Verification items for the finished model (mm, model axes). A direction names the side the tool comes from. Give positions to 0.01 mm unless a question says otherwise; leave off trailing zeros. Write each loop counter-clockwise with the first axis right and the second up, starting at its lowest first coordinate (ties: lowest second). Pieces come first, ordered by that corner, then holes. Notation, with made-up numbers: (10, -8.75) - (17, -8.75) arc R23 cw to (17, 27.25) - close; hole circle Ø7 at (54.5, -19). An arc over 180 degrees is marked (long way). Put each result on its own line as item: value.
from build123d import *

# Parameters (mm, degrees)
SKETCH1_R           = 30
SKETCH1_R_2         = 12
SKETCH1_R_3         = 20
BOSS_EXTRUDE1_DEPTH = 50
FILLET1_R           = 6
FILLET2_R           = 5


with BuildPart() as part:
    # Sketch1 → Boss-Extrude1 (new body)
    with BuildSketch(Plane.XY):
        with BuildLine():
            Line((0, 0), (168, 0))
            Line((168, 0), (168, 24))
            Line((168, 24), (134, 24))
            Line((134, 24), (134, 81.030415331))
            ThreePointArc((134, 81.030415331), (152.77498914, 93.98034061), (160, 115.613648263))
            ThreePointArc((160, 115.613648263), (155.780100416, 140.585976635), (143.589021465, 162.785128215))
            ThreePointArc((143.589021465, 162.785128215), (126.074856949, 198.422570769), (124.838141772, 238.111911984))
            ThreePointArc((124.838141772, 238.111911984), (84, 287.13508695), (43.161858228, 238.111911984))
            ThreePointArc((43.161858228, 238.111911984), (41.925143051, 198.422570769), (24.410978535, 162.785128215))
            ThreePointArc((24.410978535, 162.785128215), (12.219899584, 140.585976635), (8, 115.613648263))
            ThreePointArc((8, 115.613648263), (15.22501086, 93.98034061), (34, 81.030415331))
            Line((34, 81.030415331), (34, 24))
            Line((34, 24), (0, 24))
            Line((0, 24), (0, 0))
        make_face()
        with Locations((84, 52)):
            Circle(SKETCH1_R, mode=Mode.SUBTRACT)
        with Locations((84, 115.613648263)):
            Circle(SKETCH1_R_2, mode=Mode.SUBTRACT)
        with Locations((84, 245.613648263)):
            Circle(SKETCH1_R_3, mode=Mode.SUBTRACT)
        with BuildLine():
            ThreePointArc((110, 115.613648263), (84, 141.613648263), (58, 115.613648263))
            ThreePointArc((58, 115.613648263), (44, 101.613648263), (30, 115.613648263))
            ThreePointArc((30, 115.613648263), (84, 169.613648263), (138, 115.613648263))
            ThreePointArc((138, 115.613648263), (124, 101.613648263), (110, 115.613648263))
        make_face(mode=Mode.SUBTRACT)
    extrude(amount=BOSS_EXTRUDE1_DEPTH)

    # Fillet1
    fillet1_edges = [part.edges().sort_by_distance(p)[0] for p in [
        (34, 24, 25),
        (134, 24, 25),
    ]]
    fillet(fillet1_edges, radius=FILLET1_R)

    # Fillet2
    fillet2_edges = [part.edges().sort_by_distance(p)[0] for p in [
        (34, 81.030415331, 25),
        (134, 81.030415331, 25),
    ]]
    fillet(fillet2_edges, radius=FILLET2_R)


solid = part.part
Q1. Scan lines: line 1 along Y through (x, z) = (84, 35); line 2 along X through (y, z) = (51, 43); line 3 along Y through (x, z) = (106, 26.5). Record each from-to range of solid material in increasing order.
Answers follow:
line 1: y = 0 to 22, 82 to 103.61, 127.61 to 141.61, 169.61 to 225.61, 265.61 to 287.14
line 2: x = 34 to 54.02, 113.98 to 134
line 3: y = 0 to 31.6, 72.4 to 129.47, 164.93 to 280.83
Q2. Set-up check for faces 5 (the face through (32.196, 25.711, 25.35)), 6 (the face through (84.572, 141.607, 24.65)), 7 (the face through (135.804, 25.711, 25.35)): record each of +Z, -Z, +X, -X, +Y, -Y from which the full face is reachable in a straight line by a thin tool's end or side.
Answers follow:
face 5: +Z, -Z, -X
face 6: +Z, -Z
face 7: +Z, -Z, +X
Q3. Section check C-C, the plane z = 15. Record the cut outline in (x, y).
Answers follow:
outline: (0, 0) - (168, 0) - (168, 24) - (140, 24) arc R6 cw to (134, 30) - (134, 77.46) arc R5 cw to (137.17, 82.11) arc R36 ccw to (160, 115.61) arc R76 ccw to (143.59, 162.79) arc R94 cw to (124.84, 238.11) arc R41.52 ccw (long way) to (43.16, 238.11) arc R94 cw to (24.41, 162.79) arc R76 ccw to (8, 115.61) arc R36 ccw to (30.83, 82.11) arc R5 cw to (34, 77.46) - (34, 30) arc R6 cw to (28, 24) - (0, 24) - close; hole (30, 115.61) arc R14 ccw to (58, 115.61) arc R26 cw to (110, 115.61) arc R14 ccw to (138, 115.61) arc R54 ccw to start; hole circle Ø60 at (84, 52); hole circle Ø40 at (84, 245.61); hole circle Ø24 at (84, 115.61)
Q4. Section check A-A, the plane x = 84. Record the cut outline in (y, z), plus the area to 3 significant figures.
Answers follow:
outline: (0, 0) - (22, 0) - (22, 50) - (0, 50) - close; (82, 0) - (103.61, 0) - (103.61, 50) - (82, 50) - close; (127.61, 0) - (141.61, 0) - (141.61, 50) - (127.61, 50) - close; (169.61, 0) - (225.61, 0) - (225.61, 50) - (169.61, 50) - close; (265.61, 0) - (287.14, 0) - (287.14, 50) - (265.61, 50) - close
area: 6,760 mm2
Q5. Go/stop test with flat-tipped pins: pin 1 Ø23.5 at (y, z) = (59, 14.5) entering from +X; pin 2 Ø8 at (y, z) = (181.5, 38) entering from -X; pin 3 Ø4 at (x, z) = (72.5, 34.5) entering from +Y. Record where each tip stops, or that it passes through.
Answers follow:
pin 1: stops at x = 134
pin 2: stops at x = 33.97
pin 3: stops at y = 286.03
Q6. Section check B-B, the plane y = 248.5. Record the cut outline in (x, z), plus the area to 3 significant figures.
Answers follow:
outline: (42.58, 0) - (64.21, 0) - (64.21, 50) - (42.58, 50) - close; (103.79, 0) - (125.42, 0) - (125.42, 50) - (103.79, 50) - close
area: 2,160 mm2
Q7. Release check for a two-part mould opening along Y. For faces 1 (the face through (64, 114, 0)), 2 (the face through (126.21, 197.88, 24.65)), 3 (the face through (12.338, 140.922, 24.65)), 4 (the face through (134, 53, 25)) record: released by +Y, released by -Y, zero draft, split by the parting line, or undercut.
Answers follow:
face 1: zero draft
face 2: undercut
face 3: released by +Y
face 4: undercut
Q8. Section check D-D, the plane y = 67.5. Record the cut outline in (x, z), plus the area to 3 significant figures.
Answers follow:
outline: (34, 0) - (58.31, 0) - (58.31, 50) - (34, 50) - close; (109.69, 0) - (134, 0) - (134, 50) - (109.69, 50) - close
area: 2,430 mm2
